from build123d import *

# Parameters (mm, degrees)
SKETCH1_R           = 3.85
SKETCH1_R_2         = 2.25
BOSS_EXTRUDE1_DEPTH = 3
FILLET1_R           = 2
SKETCH2_W           = 35.37250713
SKETCH2_H           = 42.722638482
CUT_EXTRUDE1_DEPTH  = 10
FILLET2_R           = 2


with BuildPart() as part:
    # Sketch1 → Boss-Extrude1 (new body)
    with BuildSketch(Plane(origin=(0, 0, 0), x_dir=(1, 0, 0), z_dir=(0, 1, 0))):
        Polygon((-29, -12), (29, -12), (29, -6), (21.6, -6), (21.6, 6), (29, 6), (29, 12), (-29, 12), align=None)
        Circle(SKETCH1_R, mode=Mode.SUBTRACT)
        with Locations((23.8, 9)):
            Circle(SKETCH1_R_2, mode=Mode.SUBTRACT)
        with Locations((23.8, -9)):
            Circle(SKETCH1_R_2, mode=Mode.SUBTRACT)
        Polygon((-21.75, -6.129437252), (-23.1, -6.129437252), (-23.1, -4.779437252), (-24.9, -4.779437252), (-24.9, -6.129437252), (-26.25, -6.129437252), (-26.25, -7.929437252), (-24.9, -7.929437252), (-24.9, -9.279437252), (-23.1, -9.279437252), (-23.1, -7.929437252), (-21.75, -7.929437252), align=None, mode=Mode.SUBTRACT)
        Polygon((-23.1, 6.129437252), (-21.75, 6.129437252), (-21.75, 7.929437252), (-23.1, 7.929437252), (-23.1, 9.279437252), (-24.9, 9.279437252), (-24.9, 7.929437252), (-26.25, 7.929437252), (-26.25, 6.129437252), (-24.9, 6.129437252), (-24.9, 4.779437252), (-23.1, 4.779437252), align=None, mode=Mode.SUBTRACT)
    extrude(amount=BOSS_EXTRUDE1_DEPTH)

    # Fillet1
    fillet1_edges = [part.edges().sort_by_distance(p)[0] for p in [
        (29, 1.5, -6),
        (21.6, 1.5, -6),
        (21.6, 1.5, 6),
        (29, 1.5, 6),
        (29, 1.5, 12),
        (-29, 1.5, 12),
        (-29, 1.5, -12),
        (29, 1.5, -12),
    ]]
    fillet(fillet1_edges, radius=FILLET1_R)

    # Sketch2 → Cut-Extrude1 (cut)
    with BuildSketch(Plane(origin=(0, 3, 0), x_dir=(1, 0, 0), z_dir=(0, 1, 0))):
        with Locations((29.686253565, -0.298599086)):
            Rectangle(SKETCH2_W, SKETCH2_H)
    extrude(amount=-CUT_EXTRUDE1_DEPTH, mode=Mode.SUBTRACT)

    # Fillet2
    fillet2_edges = [part.edges().sort_by_distance(p)[0] for p in [
        (12, 1.5, 12),
        (12, 1.5, -12),
    ]]
    fillet(fillet2_edges, radius=FILLET2_R)


solid = part.part
Geometry check sheet. Reference: the model listing, model coordinates, mm. A direction names the side the tool comes from. Coordinates: 2 decimals unless noted, no trailing zeros. Order: outer loops, then holes, each group sorted by start corner. A loop starts at its lowest first (then second) coordinate and runs counter-clockwise, first axis right, second up. Notation, with made-up numbers: M 23.5,-32.75 L 73.5,-32.75 A17 ccw 73.5,-8.75 Z; hole C 57.5,70.5 d4. An arc over 180 degrees is marked long. Use CSV: the item, a comma, the result in double quotes.
Item 1: Cross-section at B-B on z = 0. Record the cut outline in (x, y), then the cut area to 3 significant figures.
Returned:
outline,"M -29,0 L -3.85,0 L -3.85,3 L -29,3 Z; M 3.85,0 L 12,0 L 12,3 L 3.85,3 Z"
area,"99.9 mm2"
Item 2: Mould release check, pull along Z, two halves, no side actions. Record for faces 1 (the flat face through (-26, 1, 7.929)), 2 (the flat face through (-9, 0, 0)), 3 (the flat face through (-9, 1, 12)): pulls with the +Z half, pulls with the -Z half, needs draft (parallel to the pull), parting line crosses it, or undercut.
Returned:
face 1,"undercut"
face 2,"needs draft"
face 3,"pulls with the +Z half"
Item 3: Gauge pin test, flat end, axial feed: pin 1 Ø1 at (x, z) = (-12, 6) entering from -Y. Record the tip position at first contact, or that the pin passes through.
Returned:
pin 1,"stops at y = 0"
Item 4: Tool access check on faces 4 (the flat face through (-9, 3, 0)), 5 (the flat face through (-24, 1, 4.779)). Record the directions out of +Z, -Z, +X, -X, +Y, -Y that give a thin tool (end or side, any length) a straight path to the whole face; none if there is none.
Returned:
face 4,"+Z, -Z, +X, -X, +Y"
face 5,"+Y, -Y"
Item 5: Thickness scan on line 1 along X through (y, z) = (1.95, 0); line 2 along X through (y, z) = (2.8, 6.5); line 3 along Z through (x, y) = (0, 1.3). Record the ranges inside material, lowest first.
Returned:
line 1,"x = -29 to -3.85, 3.85 to 12"
line 2,"x = -29 to -26.25, -21.75 to 12"
line 3,"z = -12 to -3.85, 3.85 to 12"
Item 6: Cross-section at A-A on x = 0. Record the cut outline in (y, z), then the cut area to 3 significant figures.
Returned:
outline,"M 0,-12 L 3,-12 L 3,-3.85 L 0,-3.85 Z; M 0,3.85 L 3,3.85 L 3,12 L 0,12 Z"
area,"48.9 mm2"
Item 7: Cross-section at C-C on y = 1.9. Give the number of separate pieces and of enclosed holes in the cut face, then the cut area to 3 significant figures.
Returned:
separate pieces,"1"
enclosed holes,"3"
area,"908 mm2"
